from build123d import *

# Parameters (mm, degrees)
F1_DEPTH = 1
F2_DEPTH = 25


with BuildPart() as f1:
    # F0 (on Front) → F1 (new body)
    with BuildSketch(Plane.XZ):
        with BuildLine():
            ThreePointArc((99.4907408065, -33.5647507629), (103.6135314153, -17.0069429252), (105, 0))
            ThreePointArc((105, 0), (103.7977584549, 15.8437792124), (100.2185649575, 31.3247384325))
            ThreePointArc((100.2185649575, 31.3247384325), (85.6336425012, 60.7608366629), (62.6663022671, 84.2492407097))
            ThreePointArc((62.6663022671, 84.2492407097), (33.5647485771, 99.4907415439), (1.1776435614, 104.9933957716))
            ThreePointArc((1.1776435614, 104.9933957716), (-31.3247392722, 100.218564695), (-60.7608381292, 85.6336414608))
            ThreePointArc((-60.7608381292, 85.6336414608), (-84.2492404255, 62.6663026493), (-99.4907409959, 33.5647502014))
            ThreePointArc((-99.4907409959, 33.5647502014), (-104.9933957718, 1.1776435403), (-100.2185647541, -31.3247390832))
            ThreePointArc((-100.2185647541, -31.3247390832), (-85.6336424849, -60.7608366859), (-62.6663027691, -84.2492403363))
            ThreePointArc((-62.6663027691, -84.2492403363), (-33.5647485613, -99.4907415492), (-1.1776429024, -104.9933957789))
            ThreePointArc((-1.1776429024, -104.9933957789), (31.3247396024, -100.2185645918), (60.7608381561, -85.6336414417))
            ThreePointArc((60.7608381561, -85.6336414417), (84.2492402585, -62.6663028738), (99.4907408065, -33.5647507629))
        make_face()
        with BuildLine():
            ThreePointArc((-60.7608381292, 85.6336414608), (-31.3247392722, 100.218564695), (1.1776435614, 104.9933957716))
            Line((1.1776435614, 104.9933957716), (-32.9367799888, 105.3760349567))
            Line((-32.9367799888, 105.3760349567), (-60.7608381292, 85.6336414608))
        make_face()
    extrude(amount=F1_DEPTH)

    # F0 (on Front) + F1_face (on face) → F2 (join)
    with BuildSketch(Plane.XZ):
        with BuildLine():
            ThreePointArc((99.4907408065, -33.5647507629), (103.6135314153, -17.0069429252), (105, 0))
            ThreePointArc((105, 0), (103.7977584549, 15.8437792124), (100.2185649575, 31.3247384325))
            ThreePointArc((100.2185649575, 31.3247384325), (85.6336425012, 60.7608366629), (62.6663022671, 84.2492407097))
            ThreePointArc((62.6663022671, 84.2492407097), (33.5647485771, 99.4907415439), (1.1776435614, 104.9933957716))
            ThreePointArc((1.1776435614, 104.9933957716), (-31.3247392722, 100.218564695), (-60.7608381292, 85.6336414608))
            ThreePointArc((-60.7608381292, 85.6336414608), (-84.2492404255, 62.6663026493), (-99.4907409959, 33.5647502014))
            ThreePointArc((-99.4907409959, 33.5647502014), (-104.9933957718, 1.1776435403), (-100.2185647541, -31.3247390832))
            ThreePointArc((-100.2185647541, -31.3247390832), (-85.6336424849, -60.7608366859), (-62.6663027691, -84.2492403363))
            ThreePointArc((-62.6663027691, -84.2492403363), (-33.5647485613, -99.4907415492), (-1.1776429024, -104.9933957789))
            ThreePointArc((-1.1776429024, -104.9933957789), (31.3247396024, -100.2185645918), (60.7608381561, -85.6336414417))
            ThreePointArc((60.7608381561, -85.6336414417), (84.2492402585, -62.6663028738), (99.4907408065, -33.5647507629))
        make_face()
        with BuildLine():
            ThreePointArc((100.2185649575, 31.3247384325), (103.7977584549, 15.8437792124), (105, 0))
            ThreePointArc((105, 0), (103.6135314153, -17.0069429252), (99.4907408065, -33.5647507629))
            Line((99.4907408065, -33.5647507629), (110.3965894634, -1.2382463674))
            Line((110.3965894634, -1.2382463674), (100.2185649575, 31.3247384325))
        make_face()
        with BuildLine():
            ThreePointArc((62.6663022671, 84.2492407097), (85.6336425012, 60.7608366629), (100.2185649575, 31.3247384325))
            Line((100.2185649575, 31.3247384325), (90.0405399504, 63.8877248356))
            Line((90.0405399504, 63.8877248356), (62.6663022671, 84.2492407097))
        make_face()
        with BuildLine():
            Line((88.5848940435, -65.8912495444), (99.4907408065, -33.5647507629))
            ThreePointArc((99.4907408065, -33.5647507629), (84.2492402585, -62.6663028738), (60.7608381561, -85.6336414417))
            Line((60.7608381561, -85.6336414417), (88.5848940435, -65.8912495444))
        make_face()
        with BuildLine():
            ThreePointArc((1.1776435614, 104.9933957716), (33.5647485771, 99.4907415439), (62.6663022671, 84.2492407097))
            Line((62.6663022671, 84.2492407097), (35.2920645417, 104.6107566152))
            Line((35.2920645417, 104.6107566152), (1.1776435614, 104.9933957716))
        make_face()
        with BuildLine():
            Line((32.9367799888, -105.3760349567), (60.7608381561, -85.6336414417))
            ThreePointArc((60.7608381561, -85.6336414417), (31.3247396024, -100.2185645918), (-1.1776429024, -104.9933957789))
            Line((-1.1776429024, -104.9933957789), (32.9367799888, -105.3760349567))
        make_face()
        with BuildLine():
            ThreePointArc((-60.7608381292, 85.6336414608), (-31.3247392722, 100.218564695), (1.1776435614, 104.9933957716))
            Line((1.1776435614, 104.9933957716), (-32.9367799888, 105.3760349567))
            Line((-32.9367799888, 105.3760349567), (-60.7608381292, 85.6336414608))
        make_face()
        with BuildLine():
            Line((-35.2920645417, -104.6107566152), (-1.1776429024, -104.9933957789))
            ThreePointArc((-1.1776429024, -104.9933957789), (-33.5647485613, -99.4907415492), (-62.6663027691, -84.2492403363))
            Line((-62.6663027691, -84.2492403363), (-35.2920645417, -104.6107566152))
        make_face()
        with BuildLine():
            ThreePointArc((-99.4907409959, 33.5647502014), (-84.2492404255, 62.6663026493), (-60.7608381292, 85.6336414608))
            Line((-60.7608381292, 85.6336414608), (-88.5848940435, 65.8912495444))
            Line((-88.5848940435, 65.8912495444), (-99.4907409959, 33.5647502014))
        make_face()
        with BuildLine():
            Line((-90.0405399504, -63.8877248356), (-62.6663027691, -84.2492403363))
            ThreePointArc((-62.6663027691, -84.2492403363), (-85.6336424849, -60.7608366859), (-100.2185647541, -31.3247390832))
            Line((-100.2185647541, -31.3247390832), (-90.0405399504, -63.8877248356))
        make_face()
        with BuildLine():
            ThreePointArc((-100.2185647541, -31.3247390832), (-104.9933957718, 1.1776435403), (-99.4907409959, 33.5647502014))
            Line((-99.4907409959, 33.5647502014), (-110.3965894634, 1.2382463674))
            Line((-110.3965894634, 1.2382463674), (-100.2185647541, -31.3247390832))
        make_face()
    with BuildSketch(Plane(origin=(-0.1080602071, -1, 0.3457215964), x_dir=(1, 0, 0), z_dir=(0, -1, 0))):
        with BuildLine():
            Line((1.2857037684, 104.6476741752), (-32.8287197817, 105.0303133603))
            Line((-32.8287197817, 105.0303133603), (-60.6527779221, 85.2879198644))
            ThreePointArc((-60.6527779221, 85.2879198644), (31.4327994792, -100.5642862914), (1.2857037684, 104.6476741752))
        make_face()
    extrude(amount=F2_DEPTH)


solid = f1.part
Read the model definition and answer for the solid it produces. Units are mm, in the model's axes. A direction names the side the tool comes from. Round coordinates to 2 decimals unless told otherwise and drop trailing zeros. Loops run counter-clockwise (first coordinate to the right, second up) from the corner with the lowest first, then second, coordinate; pieces in that order, holes last. Notation, with made-up numbers: (-30.5, 46) - (-9.5, 46) arc R23 ccw to (-9.5, 57) - close; hole circle Ø6 at (-4.75, 25.5). An arc over 180 degrees is marked (long way). One line per question, with ' | ' between items. Start each with the question number.
Q1. Section C-C on y = -6.25 is taken. Give the vertices of the cut face in (x, z), plus the area to 3 significant figures.
Q2. Section B-B on z = 11 is taken. Give the vertices of the cut face in (x, y).
Q3. Flat-ended cylindrical pins translate along their axes: pin 1 (3.5 mm diameter, centred on x = -106, z = -13.5, fed in from -Y); pin 2 (1 mm diameter, centred on x = 16, y = -21, fed in from -Z); pin 3 (2 mm diameter, centred on y = -3.5, z = 29.5, fed in from -X). Find the tip coordinate at first contact, or state that the pin passes through.
Q4. Find the intervals of material crossed by L1, parallel to Z at x = -3, y = -7.25; L2, parallel to Z at x = 54.5, y = -9.5; L3, parallel to X at y = -19.25, z = 15, in increasing order.
Q5. Section A-A on x = 84.5 is taken. Give the vertices of the cut face in (y, z).
Q6. For faces 1 (the flat face through (-86, -25, 64)), 2 (the flat face through (-86, -25, -62)), 3 (the cylindrical face through (27.33, -25.49, -101.38)), 4 (the flat face through (34, -25, 101)), determine the directions among +Z, -Z, +X, -X, +Y, -Y from which every point of the face is accessible in a straight line to the end or side of a thin tool.
Established:
1) outline: (-110.4, 1.24) - (-90.04, -63.89) - (-35.29, -104.61) - (32.94, -105.38) - (88.58, -65.89) - (110.4, -1.24) - (90.04, 63.89) - (35.29, 104.61) - (-32.94, 105.38) - (-88.58, 65.89) - close | area: 35,800 mm²
2) outline: (-107.1, -25) - (-104.42, -25) - (-104.42, -26) - (104.42, -26) - (104.42, -25) - (106.57, -25) - (106.57, 0) - (-107.1, 0) - close
3) pin 1: y = -25 | pin 2: z = -105.19 | pin 3: x = -101.2
4) L1: -104.97 to 105.04 | L2: -90.08 to 90.32 | L3: -105.75 to 105.32
5) outline: (-26, -62.33) - (-25, -62.33) - (-25, -68.79) - (0, -68.79) - (0, 68.01) - (-25, 68.01) - (-25, 62.33) - (-26, 62.33) - close
6) face 1: +Z, -X, -Y | face 2: -Z, -X, -Y | face 3: -Y | face 4: +Z, +X, -Y
